Read the model definition and answer for the solid it produces. Units are mm, in the model's axes. A direction names the side the tool comes from. Coordinates: 2 decimals unless noted, no trailing zeros. Loops run counter-clockwise (first coordinate to the right, second up) from the corner with the lowest first, then second, coordinate; pieces in that order, holes last. Notation, with made-up numbers: (16.5, 65) -> (33.5, 65) arc R27 cw to (33.5, 89) -> close; hole circle Ø9 at (42, 36.5). An arc over 180 degrees is marked (long way). Answer as a JSON object with one key per item and string values. Group by question number.
Q1. The part is cut by section C-C on y = -15. State how many separate pieces and enclosed holes the cut face has, and give its area (3 significant figures).
Q2. For faces 4 (the flat face through (-42, 19.05, 42)), 5 (the cylindrical face through (0.72, -14.29, 67.51)), determine the directions among +Z, -Z, +X, -X, +Y, -Y from which every point of the face is accessible in a straight line to the end or side of a thin tool.
Q3. The part is cut by section B-B on y = 11. Write down the section's boundary in (x, z) (3 decimals).
Q4. The part is cut by section A-A on x = 0. Write down the section's boundary in (y, z).
Q5. Determine the mould class of faces 1 (the flat face through (-54, -19.05, 24)), 2 (the cylindrical face through (59.68, 5.03, -36.68)), 3 (the cylindrical face through (-55.8, 0.2, 60.8)) for opening direction X: released by +X, released by -X, zero draft, split by the parting line, or undercut.
Q6. Straight lines are drawn through the part: line 1 along X through (y, z) = (14.5, 11); line 2 along Z through (x, y) = (8, -15); line 3 along Z through (x, y) = (-31.5, 17.5). For each, find the intervals that lie inside material, in ascending order. Write a range as [from, to].
Q7. Each of these flat-tipped pins is pushed along its axis until it touches: P1, Ø12, axis at y = -8, z = 65.5, coming from the +X side; P2, Ø5.5, axis at x = -65.5, z = -34, coming from the -Y side; P3, Ø4, axis at y = -8.5, z = -7, coming from the -X side; P4, Ø1, axis at x = -63.5, z = -40, coming from the -Y side. Where does it stop, or does it pass through?
from build123d import *

# Parameters (mm, degrees)
SKETCH1_W                                        = 38.1
SKETCH1_H                                        = 25.3746
CBORE_FOR_1_4_SOCKET_HEAD_CAP_SCREW1_D           = 7.1374
CBORE_FOR_1_4_SOCKET_HEAD_CAP_SCREW1_DEPTH       = 38.1
CBORE_FOR_1_4_SOCKET_HEAD_CAP_SCREW1_CBORE_D     = 11.1252
CBORE_FOR_1_4_SOCKET_HEAD_CAP_SCREW1_CBORE_DEPTH = 9.652
CBORE_FOR_1_4_SOCKET_HEAD_CAP_SCREW1_TIP         = 2.144291291
F_3_8_16_TAPPED_HOLE2_D                          = 7.9375
F_3_8_16_TAPPED_HOLE2_DEPTH                      = 25.4
F_3_8_16_TAPPED_HOLE2_TIP                        = 2.384665582
CHAMFER1_SIZE                                    = 1.524


with BuildPart() as part:
    # Sketch1 → Revolve1 (revolve)
    with BuildSketch(Plane(origin=(0, 0, 0), x_dir=(0, 1, 0), z_dir=(0, 0, 1)), mode=Mode.PRIVATE) as revolve1_sk:
        with Locations((0, 69.8373)):
            Rectangle(SKETCH1_W, SKETCH1_H)
    revolve(revolve1_sk.sketch.rotate(Axis((0, -44.45, 0), (0, 1, 0)), 270), axis=Axis((0, -44.45, 0), (0, 1, 0)))

    # CBORE for 1/4 Socket Head Cap Screw1
    with Locations(Plane(origin=(0, -19.05, 0), x_dir=(-1, 0, 0), z_dir=(0, -1, 0))):
        with Locations((0, -73.025), (-63.246, 36.5252), (63.246, 36.5252)):
            CounterBoreHole(CBORE_FOR_1_4_SOCKET_HEAD_CAP_SCREW1_D / 2, CBORE_FOR_1_4_SOCKET_HEAD_CAP_SCREW1_CBORE_D / 2, CBORE_FOR_1_4_SOCKET_HEAD_CAP_SCREW1_CBORE_DEPTH, depth=CBORE_FOR_1_4_SOCKET_HEAD_CAP_SCREW1_DEPTH)
            with Locations((0, 0, -(CBORE_FOR_1_4_SOCKET_HEAD_CAP_SCREW1_DEPTH + CBORE_FOR_1_4_SOCKET_HEAD_CAP_SCREW1_TIP / 2))):  # 118° drill point
                Cone(0, CBORE_FOR_1_4_SOCKET_HEAD_CAP_SCREW1_D / 2, CBORE_FOR_1_4_SOCKET_HEAD_CAP_SCREW1_TIP, mode=Mode.SUBTRACT)

    # 3/8-16 Tapped Hole2
    with Locations(Plane(origin=(0, -19.05, 0), x_dir=(-1, 0, 0), z_dir=(0, -1, 0))):
        with Locations((-69.85, 0), (69.85, 0)):
            Hole(F_3_8_16_TAPPED_HOLE2_D / 2, depth=F_3_8_16_TAPPED_HOLE2_DEPTH)
            with Locations((0, 0, -(F_3_8_16_TAPPED_HOLE2_DEPTH + F_3_8_16_TAPPED_HOLE2_TIP / 2))):  # 118° drill point
                Cone(0, F_3_8_16_TAPPED_HOLE2_D / 2, F_3_8_16_TAPPED_HOLE2_TIP, mode=Mode.SUBTRACT)

    # Chamfer1
    chamfer1_edges = [part.edges().sort_by_distance(p)[0] for p in [
        (0, -19.05, 57.15),
        (0, 19.05, 57.15),
        (0, 19.05, 82.5246),
        (0, -19.05, 82.5246),
    ]]
    chamfer(chamfer1_edges, length=CHAMFER1_SIZE)


solid = part.part
Final values:
{
 "1": {"separate pieces": "1", "enclosed holes": "6", "area": "10,700 mm2"},
 "2": {"face 4": "+Z, -Z, +X, -X, +Y", "face 5": "-Y"},
 "3": {"outline": "circle Ø165.049 at (0, 0); hole circle Ø7.137 at (-63.246, -36.525); hole circle Ø114.3 at (0, 0); hole circle Ø7.137 at (0, 73.025); hole circle Ø7.137 at (63.246, -36.525)"},
 "4": {"outline": "(-19.05, -81) -> (-17.53, -82.52) -> (17.53, -82.52) -> (19.05, -81) -> (19.05, -58.67) -> (17.53, -57.15) -> (-17.53, -57.15) -> (-19.05, -58.67) -> close; (-19.05, 58.67) -> (-17.53, 57.15) -> (17.53, 57.15) -> (19.05, 58.67) -> (19.05, 69.46) -> (-9.4, 69.46) -> (-9.4, 67.46) -> (-19.05, 67.46) -> close; (-19.05, 78.59) -> (-9.4, 78.59) -> (-9.4, 76.59) -> (19.05, 76.59) -> (19.05, 81) -> (17.53, 82.52) -> (-17.53, 82.52) -> (-19.05, 81) -> close"},
 "5": {"face 1": "zero draft", "face 2": "undercut", "face 3": "split by the parting line"},
 "6": {"line 1": "x = [-81.79, -56.08], [56.08, 81.79]", "line 2": "z = [-82.14, -56.59], [56.59, 82.14]", "line 3": "z = [-76.28, -47.69], [47.69, 76.28]"},
 "7": {"P1": "stops at x = 57.18", "P2": "stops at y = -19.05", "P3": "stops at x = -82.37", "P4": "stops at y = -9.4"}
}
